CAD build for the part. Positions are in the model's coordinates, mm. Round coordinates to 2 decimals unless told otherwise and drop trailing zeros. Order: outer loops, then holes, each group sorted by start corner. A loop starts at its lowest first (then second) coordinate and runs counter-clockwise, first axis right, second up.
```python
from build123d import *

# Parameters (mm, degrees)
SKETCH1_W            = 254
SKETCH1_H            = 381
BOSS_EXTRUDE1_DEPTH  = 1.5875
SKETCH2_R            = 1.4732
CUT_EXTRUDE1_DEPTH   = 458.907763809
FILLET1_R            = 3.175
SKETCH5_R            = 1.4732
CUT_EXTRUDE3_DEPTH   = 458.907763809
LPATTERN1_COUNT      = 4
LPATTERN1_PITCH      = 96.8756
LPATTERN1_COUNT_DIR2 = 2
LPATTERN1_PITCH_DIR2 = 161.5948
CUT_EXTRUDE4_DEPTH   = 458.907763809


with BuildPart() as part:
    # Sketch1 → Boss-Extrude1 (new body)
    with BuildSketch(Plane.XY):
        with Locations((127, 190.5)):
            Rectangle(SKETCH1_W, SKETCH1_H)
    extrude(amount=BOSS_EXTRUDE1_DEPTH)

    # Sketch2 → Cut-Extrude1 (cut, through all)
    with BuildSketch(Plane.XY.offset(1.5875)):
        with Locations((3.81, 377.19)):
            Circle(SKETCH2_R)
        with Locations(Location((89.8652, 377.19, 0), (0, 0, 180))):
            Circle(SKETCH2_R)
        with Locations(Location((164.1348, 377.19, 0), (0, 0, 180))):
            Circle(SKETCH2_R)
        with Locations((250.19, 377.19)):
            Circle(SKETCH2_R)
        with Locations(Location((164.1348, 287.375451288, 0), (0, 0, 180))):
            Circle(SKETCH2_R)
        with Locations((3.81, 287.3756)):
            Circle(SKETCH2_R)
        with Locations((250.19, 287.3756)):
            Circle(SKETCH2_R)
        with Locations((89.8652, 287.3756)):
            Circle(SKETCH2_R)
        with Locations(Location((164.1348, 190.499990436, 0), (0, 0, 180))):
            Circle(SKETCH2_R)
        with Locations((3.81, 191.135)):
            Circle(SKETCH2_R)
        with Locations((250.19, 190.5)):
            Circle(SKETCH2_R)
        with Locations((89.8652, 190.5)):
            Circle(SKETCH2_R)
        with Locations(Location((164.1348, 93.6244, 0), (0, 0, 180))):
            Circle(SKETCH2_R)
        with Locations((3.81, 93.6244)):
            Circle(SKETCH2_R)
        with Locations((250.19, 93.6244)):
            Circle(SKETCH2_R)
        with Locations((89.8652, 93.6244)):
            Circle(SKETCH2_R)
        with Locations(Location((164.1348, 3.81, 0), (0, 0, 180))):
            Circle(SKETCH2_R)
        with Locations((3.81, 3.81)):
            Circle(SKETCH2_R)
        with Locations((250.19, 3.81)):
            Circle(SKETCH2_R)
        with Locations((89.8652, 3.81)):
            Circle(SKETCH2_R)
    extrude(amount=-CUT_EXTRUDE1_DEPTH, mode=Mode.SUBTRACT)

    # Fillet1
    fillet1_edges = [part.edges().sort_by_distance(p)[0] for p in [
        (0, 381, 0.79375),
        (254, 381, 0.79375),
        (254, 0, 0.79375),
        (0, 0, 0.79375),
    ]]
    fillet(fillet1_edges, radius=FILLET1_R)

    # Sketch5 → Cut-Extrude3 (cut, through all)
    with BuildSketch(Plane.XY.offset(1.5875)):
        with Locations((25.2476, 74.3966)):
            Circle(SKETCH5_R)
        with Locations(Location((67.1576, 74.3966, 0), (0, 0, 180))):
            Circle(SKETCH5_R)
        with Locations((67.1576, 15.9766)):
            Circle(SKETCH5_R)
        with Locations(Location((25.2476, 15.9766, 0), (0, 0, 180))):
            Circle(SKETCH5_R)
    cut_extrude3 = extrude(amount=-CUT_EXTRUDE3_DEPTH, mode=Mode.SUBTRACT)

    # LPattern1: Cut-Extrude3 4 × 2
    with Locations(*[(j * LPATTERN1_PITCH_DIR2, i * LPATTERN1_PITCH, 0) for i in range(LPATTERN1_COUNT) for j in range(LPATTERN1_COUNT_DIR2) if (i, j) != (0, 0)]):
        add(cut_extrude3, mode=Mode.SUBTRACT)

    # Sketch6 → Cut-Extrude4 (cut, through all)
    with BuildSketch(Plane.XY.offset(1.5875)):
        Polygon((295.552123895, 381), (107.714500619, 381), (107.714500619, 277.29497196), (0, 277.29497196), (0, -37.89474057), (295.552123895, -37.89474057), align=None)
    extrude(amount=-CUT_EXTRUDE4_DEPTH, mode=Mode.SUBTRACT)


solid = part.part
```
1. Cut at A-A, the plane x = 67. Write the cut outline in (y, z), and give its area (3 significant figures).
2. Mould opens along X. For faces 1 (the face through (53, 330, 0)), 2 (the face through (89.673, 288.836, 0.805)), 3 (the face through (0.91, 380.05, 0.8)) say: released by +X, released by -X, zero draft, split by the parting line, or undercut.
3. Drill centre lines: line 1 (Y direction, x = 3.81, z = 1.15); line 2 (X direction, y = 365, z = 0.55). Where is each one in solid material? Low to high.
4. Pin check, flat tip, straight feed: P1, Ø4, axis at x = 51, y = 359, coming from the -Z side. Stop position of the tip, or through.
Outcome:
1. outline: (277.29, 0) - (305.14, 0) - (305.14, 1.59) - (277.29, 1.59) - close; (308.07, 0) - (363.56, 0) - (363.56, 1.59) - (308.07, 1.59) - close; (366.49, 0) - (381, 0) - (381, 1.59) - (366.49, 1.59) - close
1. area: 155 mm2
2. face 1: zero draft
2. face 2: undercut
2. face 3: released by -X
3. line 1: y = 277.29 to 285.9, 288.85 to 375.72, 378.66 to 381
3. line 2: x = 0 to 23.77, 26.72 to 65.68, 68.63 to 107.71
4. P1: stops at z = 0
